Source: CAD feature listing. Evaluate the final solid. Frame: model axes, mm. A direction names the side the tool comes from. Round coordinates to 2 decimals unless told otherwise and drop trailing zeros. Order: outer loops, then holes, each group sorted by start corner. A loop starts at its lowest first (then second) coordinate and runs counter-clockwise, first axis right, second up. Notation, with made-up numbers: (25.25, -3.5) -> (73.25, -3.5) arc R29 ccw to (73.25, 19.5) -> close; hole circle Ø8 at (60.5, -35.75). An arc over 180 degrees is marked (long way). Write item = value, one per line. Start each with the question number.
(1) Cut plane C-C on y = -4. Return the cut outline in (x, z), then the cut area to 3 significant figures.
(2) Cut plane A-A on z = 8.25. Return the cut outline in (x, y).
(3) Ray query, line 1 (Y direction, x = 12.25, z = 5.75); line 2 (X direction, y = -2.25, z = 10.25); line 3 (Y direction, x = -0.5, z = 8). Return the intervals inside material, ascending.
(4) Cut plane B-B on x = -3. Return the cut outline in (y, z), then the cut area to 3 significant figures.
(5) Reachability of faces 1 (the face through (-2, -8, 6)), 2 (the face through (3, 1, 0)), 3 (the face through (0, 3, 15)), 4 (the face through (9, 0, 7)), 5 (the face through (8, 2, 6)) from +Z, -Z, +X, -X, +Y, -Y: full face, straight path, thin tool, end or side. Return the list, or none.
(6) Draft query along Y for faces 6 (the face through (0, -9, 7)), 7 (the face through (5, 7, 7)), 8 (the face through (2, 3, 13)). Return one class per face: released by +Y, released by -Y, zero draft, split by the parting line, or undercut.
(7) Cut plane D-D on x = 3. Return the cut outline in (y, z), then the cut area to 3 significant figures.
(8) Contact query for a flat-ended pin moving along its axis: pin 1 Ø6 at (y, z) = (-5, 12) entering from +X. Output: stop coordinate, or through.
from build123d import *

# Parameters (mm, degrees)
PAD_DEPTH    = 15
POCKET_DEPTH = 13
FILLET_R     = 0.5


with BuildPart() as part:
    # Sketch → Pad (new body)
    with BuildSketch(Plane.XY):
        Polygon((0, 0), (0, -18), (-7, -18), (-7, 7), (18, 7), (18, 0), align=None)
    extrude(amount=PAD_DEPTH)

    # Sketch001 → Pocket (cut)
    with BuildSketch(Plane.XY):
        Polygon((-2, 2), (-2, -20), (-5, -20), (-5, 5), (20, 5), (20, 2), align=None)
    extrude(amount=POCKET_DEPTH, mode=Mode.SUBTRACT)

    # Fillet
    fillet_edges = [part.edges().sort_by_distance(p)[0] for p in [
        (0, -9, 15),
        (-3.5, -18, 15),
        (-7, -5.5, 15),
        (5.5, 7, 15),
        (18, 3.5, 15),
        (9, 0, 15),
        (-7, -18, 7.5),
        (-7, 7, 7.5),
        (-7, -5.5, 0),
        (0, 0, 7.5),
        (0, -18, 7.5),
        (0, -9, 0),
        (18, 0, 7.5),
        (9, 0, 0),
        (18, 7, 7.5),
        (5.5, 7, 0),
        (-1, -18, 0),
        (-2, -18, 6.5),
        (-3.5, -18, 13),
        (-5, -18, 6.5),
        (-6, -18, 0),
        (18, 6, 0),
        (18, 5, 6.5),
        (18, 3.5, 13),
        (18, 2, 6.5),
        (18, 1, 0),
        (-2, -8, 13),
        (-5, -6.5, 13),
        (6.5, 5, 13),
        (8, 2, 13),
        (-2, -8, 0),
        (-2, 2, 6.5),
        (8, 2, 0),
    ]]
    fillet(fillet_edges, radius=FILLET_R)


solid = part.part
Evaluation:
q1.outline = (-7, 0.5) arc R0.5 ccw to (-6.5, 0) -> (-5, 0) -> (-5, 12.5) arc R0.5 cw to (-4.5, 13) -> (-2.5, 13) arc R0.5 cw to (-2, 12.5) -> (-2, 0.5) arc R0.5 ccw to (-1.5, 0) -> (-0.5, 0) arc R0.5 ccw to (0, 0.5) -> (0, 14.5) arc R0.5 ccw to (-0.5, 15) -> (-6.5, 15) arc R0.5 ccw to (-7, 14.5) -> close
q1.area = 65.8 mm^2
q2.outline = (-7, -17.5) arc R0.5 ccw to (-6.5, -18) -> (-5.5, -18) arc R0.5 ccw to (-5, -17.5) -> (-5, 5) -> (17.5, 5) arc R0.5 ccw to (18, 5.5) -> (18, 6.5) arc R0.5 ccw to (17.5, 7) -> (-6.5, 7) arc R0.5 ccw to (-7, 6.5) -> close; (-2, -17.5) arc R0.5 ccw to (-1.5, -18) -> (-0.5, -18) arc R0.5 ccw to (0, -17.5) -> (0, -0.5) arc R0.5 cw to (0.5, 0) -> (17.5, 0) arc R0.5 ccw to (18, 0.5) -> (18, 1.5) arc R0.5 ccw to (17.5, 2) -> (-1.5, 2) arc R0.5 ccw to (-2, 1.5) -> close
q3.line_1 = 0 to 2, 5 to 7
q3.line_2 = -7 to -5, -2 to 0
q3.line_3 = -18 to 2, 5 to 7
q4.outline = (-18, 13.5) arc R0.5 ccw to (-17.5, 13) -> (4.5, 13) arc R0.5 cw to (5, 12.5) -> (5, 0) -> (6.5, 0) arc R0.5 ccw to (7, 0.5) -> (7, 14.5) arc R0.5 ccw to (6.5, 15) -> (-17.5, 15) arc R0.5 ccw to (-18, 14.5) -> close
q4.area = 75.8 mm^2
q5.face_1 = -Z, -Y
q5.face_2 = -Z, +X, -X, +Y, -Y
q5.face_3 = +Z, +X, -X, +Y, -Y
q5.face_4 = +Z, -Z, +X, -Y
q5.face_5 = -Z, +X
q6.face_6 = zero draft
q6.face_7 = released by +Y
q6.face_8 = undercut
q7.outline = (0, 0.5) arc R0.5 ccw to (0.5, 0) -> (1.5, 0) arc R0.5 ccw to (2, 0.5) -> (2, 12.5) arc R0.5 cw to (2.5, 13) -> (4.5, 13) arc R0.5 cw to (5, 12.5) -> (5, 0) -> (6.5, 0) arc R0.5 ccw to (7, 0.5) -> (7, 14.5) arc R0.5 ccw to (6.5, 15) -> (0.5, 15) arc R0.5 ccw to (0, 14.5) -> close
q7.area = 65.8 mm^2
q8.pin_1 = 0
